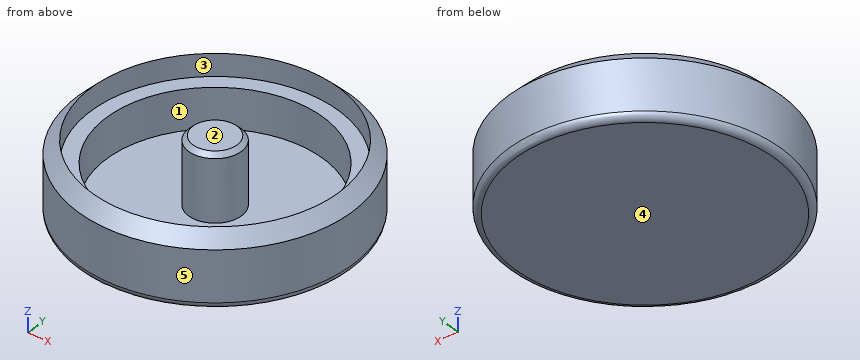
from build123d import *

# Parameters (mm, degrees)
F0_R     = 12.4
F0_R_2   = 9.8
F1_DEPTH = 3.6
F2_R     = 12.4
F2_R_2   = 9.8
F3_DEPTH = 0.8
F4_R     = 12.4
F4_R_2   = 11.2
F5_DEPTH = 2
F6_R     = 0.6
F7_R     = 2.4
F8_DEPTH = 6
F9_SIZE  = 0.4


# Not quite as in the source:
# - a fillet or chamfer that OpenCascade refuses, or shapes differently, is made with other operations: its cross-section is extruded or revolved along the edge and cut away or added


with BuildPart() as f1:
    # F0 (on Top) → F1 (new body)
    with BuildSketch(Plane.XY):
        Circle(F0_R)
        Circle(F0_R_2, mode=Mode.SUBTRACT)
    extrude(amount=F1_DEPTH)

    # F2 (on face) → F3 (join)
    with BuildSketch(Plane(origin=(0, 0, 0), x_dir=(1, 0, 0), z_dir=(0, 0, -1))):
        Circle(F2_R)
        Circle(F2_R_2, mode=Mode.SUBTRACT)
        Circle(F2_R_2)
    extrude(amount=F3_DEPTH)

    # F4 (on face) → F5 (join)
    with BuildSketch(Plane.XY.offset(3.6)):
        Circle(F4_R)
        Circle(F4_R_2, mode=Mode.SUBTRACT)
    extrude(amount=F5_DEPTH)

    # F6
    f6_edges = [f1.edges().sort_by_distance(p)[0] for p in [
        (-12.4, 0, -0.8),
    ]]
    fillet(f6_edges, radius=F6_R)

    # F7 (on face) → F8 (join)
    with BuildSketch(Plane.XY):
        Circle(F7_R)
    extrude(amount=F8_DEPTH)

    # F9
    f9_edges = [f1.edges().sort_by_distance(p)[0] for p in [
        (-2.4, 0, 6),
    ]]
    chamfer(f9_edges, length=F9_SIZE)

    # F10: chamfer of 1.2 on 1 edges, made by hand

    # F10_s1 → F10_t2 (revolve, cut)
    with BuildSketch(Plane.XZ):
        Polygon((11.2, 5.6), (12.4, 4.4), (12.4, 5.6), align=None)
    revolve(axis=Axis((0, 0, 5.6), (0, 0, 1)), mode=Mode.SUBTRACT)


solid = f1.part
Geometry check sheet. Reference: the model listing, model coordinates, mm. Face numbers are marked on the shaded views. A direction names the side the tool comes from. Round coordinates to 2 decimals unless told otherwise and drop trailing zeros. Loops run counter-clockwise (first coordinate to the right, second up) from the corner with the lowest first, then second, coordinate; pieces in that order, holes last. Notation, with made-up numbers: (15.5, 6) - (64.5, 6) arc R35 ccw to (64.5, 43) - close; hole circle Ø1 at (-7.5, -8.75). An arc over 180 degrees is marked (long way). Answer as CSV lines item,"result".
(1) Depth check by flat-ended pin: pin 1 Ø2 at (x, z) = (-9.5, 4.5) entering from +Y; pin 2 Ø1 at (x, z) = (-1, 0.5) entering from -Y; pin 3 Ø8 at (x, y) = (-6, 9.5) entering from +Z. Enter the tip coordinate at first touch or a pass-through.
Output values:
pin 1,"stops at y = 9.02"
pin 2,"stops at y = -12.39"
pin 3,"stops at z = 5.6"
(2) Cross-section at A-A, the plane z = 4. Enter the section's corners in (x, y).
Output values:
outline,"circle Ø24.8 at (0, 0); circle Ø4.8 at (0, 0); hole circle Ø22.4 at (0, 0)"
(3) Set-up check for the marked faces 1 and 2: record each of +Z, -Z, +X, -X, +Y, -Y from which the full face is reachable in a straight line by a thin tool's end or side.
Output values:
face 1,"+Z"
face 2,"+Z, +X, -X, +Y, -Y"
(4) Release check for a two-part mould opening along X. For the marked faces 3, 4 and 5 record: released by +X, released by -X, zero draft, split by the parting line, or undercut.
Output values:
face 3,"undercut"
face 4,"zero draft"
face 5,"split by the parting line"
(5) Cross-section at B-B, the plane y = 0. Enter the section's corners in (x, z).
Output values:
outline,"(-12.4, -0.2) arc R0.6 ccw to (-11.8, -0.8) - (11.8, -0.8) arc R0.6 ccw to (12.4, -0.2) - (12.4, 4.4) - (11.2, 5.6) - (11.2, 3.6) - (9.8, 3.6) - (9.8, 0) - (2.4, 0) - (2.4, 5.6) - (2, 6) - (-2, 6) - (-2.4, 5.6) - (-2.4, 0) - (-9.8, 0) - (-9.8, 3.6) - (-11.2, 3.6) - (-11.2, 5.6) - (-12.4, 4.4) - close"
(6) Material ranges on line 1 along Y through (x, z) = (0, 1.8); line 2 along Y through (x, z) = (0, 5.05); line 3 along Z through (x, y) = (-6.25, 7), recorded low to high.
Output values:
line 1,"y = -12.4 to -9.8, -2.4 to 2.4, 9.8 to 12.4"
line 2,"y = -11.75 to -11.2, -2.4 to 2.4, 11.2 to 11.75"
line 3,"z = -0.8 to 0"
